from build123d import *

# Parameters (mm, degrees)
SKETCH1_R           = 15.875
BOSS_EXTRUDE1_DEPTH = 20.701
SWEEP1_PROFILE_R    = 9.525
SWEEP2_PROFILE_R    = 9.525
CUT_EXTRUDE1_REACH  = 233.612
SKETCH2_R           = 12.7
SKETCH36_R          = 7.9375
CUT_EXTRUDE2_DEPTH  = 127
SKETCH37_R          = 7.9375
CUT_EXTRUDE3_DEPTH  = 127
SWEEP3_PROFILE_R    = 12.7


with BuildPart() as part:
    # Sketch1 → Boss-Extrude1 (new, symmetric)
    with BuildSketch(Plane(origin=(0, 0, 0), x_dir=(1, 0, 0), z_dir=(0, 0.34202014332566943, 0.9396926207859081))):
        with Locations(Location((0, 0, 0), (0, 0, 270))):
            Circle(SKETCH1_R)
    extrude(amount=BOSS_EXTRUDE1_DEPTH, both=True)

    # Sweep1: sweep along a path in Sketch4
    with BuildLine(Plane(origin=(0, 3.126764616, 3.726332964), x_dir=(1, 0, 0), z_dir=(0, 0.6427876096865406, 0.7660444431189771))) as sweep1_path:
        Line((-5.08, -4.081701322), (-96.768607765, 201.854283468))
    # Sweep1 profile (on start of the path) → Sweep1 (sweep)
    with BuildSketch(Plane(origin=(-5.08, 0, 6.35), x_dir=(0, 0.6427876096865406, 0.7660444431189771), z_dir=(-0.4067366430758009, 0.6998164213636971, -0.5872157010580841))):
        Circle(SWEEP1_PROFILE_R)
    sweep(path=sweep1_path.line)

    # Sweep2: sweep along a path in Sketch15
    with BuildLine(Plane(origin=(0, 3.126764616, 3.726332964), x_dir=(1, 0, 0), z_dir=(0, 0.6427876096865406, 0.7660444431189771))) as sweep2_path:
        Line((5.08, -4.081701322), (96.768607765, 201.854283468))
    # Sweep2 profile (on start of the path) → Sweep2 (sweep)
    with BuildSketch(Plane(origin=(5.08, 0, 6.35), x_dir=(0, 0.6427876096865406, 0.766044443118977), z_dir=(0.40673664307580104, 0.6998164213636969, -0.587215701058084))):
        Circle(SWEEP2_PROFILE_R)
    sweep(path=sweep2_path.line)

    # Sketch2 → Cut-Extrude1 (cut, up to next)
    with BuildSketch(Plane(origin=(0, -7.080158987, -19.452576943), x_dir=(-1, 0, 0), z_dir=(0, -0.34202014332566943, -0.9396926207859081)), mode=Mode.PRIVATE) as cut_extrude1_sk1:
        with Locations(Location((0, 0, 0), (0, 0, 90))):
            Circle(SKETCH2_R)
    cut_extrude1_tool1 = extrude(cut_extrude1_sk1.sketch, amount=-CUT_EXTRUDE1_REACH, mode=Mode.PRIVATE) & part.part
    add(cut_extrude1_tool1.solids().sort_by_distance((0, -7.080159, -19.452577))[0], mode=Mode.SUBTRACT)

    # Sketch36 → Cut-Extrude2 (cut)
    with BuildSketch(Plane(origin=(-91.012368417, 156.592603715, -131.396796022), x_dir=(0.9135454575587967, 0.3115870518309583, -0.26143489840681283), z_dir=(-0.40673664307580104, 0.6998164213636969, -0.5872157010580842))):
        with Locations(Location((-6.300922529, -4.864467561, 0), (0, 0, 270.000776077))):
            Circle(SKETCH36_R)
    extrude(amount=-CUT_EXTRUDE2_DEPTH, mode=Mode.SUBTRACT)

    # Sketch37 → Cut-Extrude3 (cut)
    with BuildSketch(Plane(origin=(91.012368417, 156.592603715, -131.396796022), x_dir=(0.9135454575587966, -0.3115870518309586, 0.261434898406813), z_dir=(0.4067366430758013, 0.699816421363697, -0.5872157010580837))):
        with Locations(Location((6.300922529, -4.864467561, 0), (0, 0, 269.999223923))):
            Circle(SKETCH37_R)
    extrude(amount=-CUT_EXTRUDE3_DEPTH, mode=Mode.SUBTRACT)

    # Sweep3: sweep along a path in Sketch40
    with BuildLine(Plane(origin=(-106.934, 0, -127), x_dir=(1, 0, 0), z_dir=(0, 0, 1))) as sweep3_path:
        Line((-62.089448271, 150.498042412), (101.994706052, 159.628680082))
        ThreePointArc((101.994706052, 159.628680082), (106.934, 159.766), (111.873293948, 159.628680082))
        Line((111.873293948, 159.628680082), (275.957448271, 150.498042412))
    # Sweep3 profile (on start of the path) → Sweep3 (sweep)
    with BuildSketch(Plane(origin=(-169.023448271, 150.498042412, -127), x_dir=(-0.0555601119023539, 0.9984553440016224, 0), z_dir=(0.9984553440016224, 0.0555601119023539, 0))):
        Circle(SWEEP3_PROFILE_R)
    sweep(path=sweep3_path.line)


solid = part.part
Read the model definition and answer for the solid it produces. Units are mm, in the model's axes. A direction names the side the tool comes from. Give positions to 0.01 mm unless a question says otherwise; leave off trailing zeros. Use a Markdown table: item, result.
Q1. Section A-A, the plane z = -51 is taken. Count the separate pieces of the cut face and the enclosed holes in it, then the cut area to 3 significant figures.
Solved:
| item | result |
|---|---|
| separate pieces | 2 |
| enclosed holes | 2 |
| area | 664 mm^2 |
Q2. Find the intervals of material crossed by line 1 along Y through (x, z) = (-62.5, -85.5); line 2 along X through (y, z) = (7.5, 15.5); line 3 along X through (y, z) = (60, -50), in increasing order.
Solved:
| item | result |
|---|---|
| line 1 | y = 94.74 to 97.49, 114.52 to 117.27 |
| line 2 | x = -15.78 to -12.58, 12.58 to 15.78 |
| line 3 | x = -50.8 to -32.54, 32.54 to 50.8 |
Q3. Each of these flat-tipped pins is pushed along its axis until it touches: pin 1 (10 mm diameter, centred on x = -43, y = 59.5, fed in from +Z); pin 2 (1.5 mm diameter, centred on y = 34.5, z = -25.5, fed in from +X); pin 3 (10 mm diameter, centred on y = 151.5, z = -112.5, fed in from +X). Where does it stop, or does it pass through?
Solved:
| item | result |
|---|---|
| pin 1 | stops at z = -29.69 |
| pin 2 | stops at x = 36.48 |
| pin 3 | stops at x = 169.31 |
Q4. A tool of negligible diameter and unlimited length cuts with its end or side. For faces 1 (the face through (90.692, 147.856, -116.397)), 2 (the face through (169.014, 150.321, -126.822)), from which of +Z, -Z, +X, -X, +Y, -Y can it reach the whole face along a straight path? Write none if from no direction.
Solved:
| item | result |
|---|---|
| face 1 | none |
| face 2 | +Z, -Z, +X, -Y |
Q5. Determine the mould class of faces 3 (the face through (13.009, 7.15, 19.427)), 4 (the face through (-169.014, 150.321, -126.822)), 5 (the face through (-90.453, 147.87, -116.397)) for opening direction Y: pulls with the +Y half, pulls with the -Y half, needs draft (parallel to the pull), parting line crosses it, or undercut.
Solved:
| item | result |
|---|---|
| face 3 | pulls with the +Y half |
| face 4 | pulls with the -Y half |
| face 5 | undercut |
